Model file for the job. Use its own axes, mm. A direction names the side the tool comes from. Round coordinates to 2 decimals unless told otherwise and drop trailing zeros. Loops run counter-clockwise (first coordinate to the right, second up) from the corner with the lowest first, then second, coordinate; pieces in that order, holes last. Notation, with made-up numbers: M 86,43.25 L 143,43.25 A37 cw 143,79.25 Z; hole C 11,16.5 d9. An arc over 180 degrees is marked long. Use a Markdown table: item, result. Add a question column.
Item 1: Tool access for faces 5 (the flat face through (-44.25, 0.49, -44.49)), 6 (the flat face through (44.25, 0.51, -31.72)): list every direction of +Z, -Z, +X, -X, +Y, -Y with a clear straight run to the whole face (end or side of a thin tool).
Item 2: Saw through at A-A on z = 9.5. Write the cut outline in (x, y).
Item 3: Wall check: L1, parallel to Z at x = -38.5, y = 0.35; L2, parallel to Z at x = -10, y = 0.7; L3, parallel to Z at x = 3, y = 0.5. Give the ranges that are in metal, low to high. Write a range as from..to.
Item 4: Saw through at D-D on x = 50. Write the cut outline in (y, z).
Item 5: Saw through at B-B on x = -16.5. Write the cut outline in (y, z).
Item 6: Saw through at C-C on y = 0.8. Give the number of separate pieces and of enclosed holes in the cut face, then the cut area to 3 significant figures.
Item 7: Two-plate mould, pull along X, no slides. Class faces 1 (the flat face through (-24.17, 0.49, 57.91)), 2 (the flat face through (23.85, 0.49, 58.04)), 3 (the flat face through (44.25, 0.51, 31.72)), 4 (the flat face through (36.74, 0.493, -42.455)): +X half, -X half, draft (parallel to the pull), parting line (faces both ways), or undercut.
Item 8: Pin check, flat tip, straight feed: P1, Ø0.5, axis at x = 51.5, y = 0.5, coming from the +Z side. Stop position of the tip, or through.
```python
from build123d import *

# Parameters (mm, degrees)
BOSS_EXTRUDE1_DEPTH = 1
SKETCH2_W           = 10
SKETCH2_H           = 10
BOSS_EXTRUDE2_DEPTH = 1
SKETCH3_R           = 1.5
BOSS_EXTRUDE3_DEPTH = 1
CHAMFER1_SIZE       = 1.5


with BuildPart() as part:
    # Sketch1 → Boss-Extrude1 (new body)
    with BuildSketch(Plane(origin=(0, 0, 0), x_dir=(1, 0, 0), z_dir=(0, 1, 0))):
        Polygon((62.75, -12.481751053), (62.75, 12.481751053), (53.19688133, 35.545019709), (35.545019709, 53.19688133), (12.481751053, 62.75), (-12.481751053, 62.75), (-35.545019709, 53.19688133), (-53.19688133, 35.545019709), (-62.75, 12.481751053), (-62.75, -12.481751053), (-53.19688133, -35.545019709), (-35.545019709, -53.19688133), (-12.481751053, -62.75), (12.481751053, -62.75), (35.545019709, -53.19688133), (53.19688133, -35.545019709), align=None)
        Polygon((56, -11.139092573), (56, 11.139092573), (47.474507641, 31.721451852), (31.721451852, 47.474507641), (11.139092573, 56), (-11.139092573, 56), (-31.721451852, 47.474507641), (-47.474507641, 31.721451852), (-56, 11.139092573), (-56, -11.139092573), (-47.474507641, -31.721451852), (-31.721451852, -47.474507641), (-11.139092573, -56), (11.139092573, -56), (31.721451852, -47.474507641), (47.474507641, -31.721451852), align=None, mode=Mode.SUBTRACT)
    extrude(amount=BOSS_EXTRUDE1_DEPTH)

    # Sketch2 → Boss-Extrude2 (add)
    with BuildSketch(Plane(origin=(0, 1, 0), x_dir=(1, 0, 0), z_dir=(0, 1, 0))):
        with Locations((0, 51)):
            Rectangle(SKETCH2_W, SKETCH2_H)
        with Locations((51, 0)):
            Rectangle(SKETCH2_W, SKETCH2_H)
        with Locations((0, -51)):
            Rectangle(SKETCH2_W, SKETCH2_H)
        with Locations((-51, 0)):
            Rectangle(SKETCH2_W, SKETCH2_H)
    extrude(amount=-BOSS_EXTRUDE2_DEPTH)

    # Sketch3 → Boss-Extrude3 (add)
    # profile 1 of 4: a face of its own
    with BuildSketch(Plane(origin=(0, 1, 0), x_dir=(1, 0, 0), z_dir=(0, 1, 0))):
        Polygon((-45.863587475, 33.332372018), (-41.620946788, 37.575012705), (-37.378306101, 33.332372018), (-41.620946788, 29.08973133), align=None)
        with Locations(Location((-41.620946788, 33.332372018, 0), (0, 0, 270))):
            Circle(SKETCH3_R, mode=Mode.SUBTRACT)
    # profile 2 of 4: a face of its own
    with BuildSketch(Plane(origin=(0, 1, 0), x_dir=(1, 0, 0), z_dir=(0, 1, 0))):
        Polygon((37.378306101, 33.332372018), (41.620946788, 29.08973133), (45.863587475, 33.332372018), (41.620946788, 37.575012705), align=None)
        with Locations(Location((41.620946788, 33.332372018, 0), (0, 0, 270))):
            Circle(SKETCH3_R, mode=Mode.SUBTRACT)
    # profile 3 of 4: a face of its own
    with BuildSketch(Plane(origin=(0, 1, 0), x_dir=(1, 0, 0), z_dir=(0, 1, 0))):
        Polygon((41.620946788, -37.575012705), (37.378306101, -33.332372018), (41.620946788, -29.08973133), (45.863587475, -33.332372018), align=None)
        with Locations(Location((41.620946788, -33.332372018, 0), (0, 0, 270))):
            Circle(SKETCH3_R, mode=Mode.SUBTRACT)
    # profile 4 of 4: a face of its own
    with BuildSketch(Plane(origin=(0, 1, 0), x_dir=(1, 0, 0), z_dir=(0, 1, 0))):
        Polygon((-37.378306101, -33.332372018), (-41.620946788, -29.08973133), (-45.863587475, -33.332372018), (-41.620946788, -37.575012705), align=None)
        with Locations(Location((-41.620946788, -33.332372018, 0), (0, 0, 270))):
            Circle(SKETCH3_R, mode=Mode.SUBTRACT)
    extrude(amount=-BOSS_EXTRUDE3_DEPTH)

    # Chamfer1
    chamfer1_edges = [part.edges().sort_by_distance(p)[0] for p in [
        (-37.378306101, 0.5, -33.332372018),
        (-41.620946788, 0.5, -29.08973133),
        (41.620946788, 0.5, -29.08973133),
        (37.378306101, 0.5, -33.332372018),
        (41.620946788, 0.5, 29.08973133),
        (37.378306101, 0.5, 33.332372018),
        (-41.620946788, 0.5, 29.08973133),
        (-37.378306101, 0.5, 33.332372018),
    ]]
    chamfer(chamfer1_edges, length=CHAMFER1_SIZE)


solid = part.part
```
Entries:
| question | item | result |
|---|---|---|
| 1 | face 5 | -Z, -X, +Y, -Y |
| 1 | face 6 | +Y, -Y |
| 2 | outline | M -62.75,0 L -56,0 L -56,1 L -62.75,1 Z; M 56,0 L 62.75,0 L 62.75,1 L 56,1 Z |
| 3 | L1 | -50.24..-40.7, -34.45..-32.21, 32.21..34.45, 40.7..50.24 |
| 3 | L2 | -62.75..-56, 56..62.75 |
| 3 | L3 | -62.75..-46, 46..62.75 |
| 4 | outline | M 0,-38.74 L 1,-38.74 L 1,-25.62 L 0,-25.62 Z; M 0,-5 L 1,-5 L 1,5 L 0,5 Z; M 0,25.62 L 1,25.62 L 1,38.74 L 0,38.74 Z |
| 5 | outline | M 0,-61.09 L 1,-61.09 L 1,-53.78 L 0,-53.78 Z; M 0,53.78 L 1,53.78 L 1,61.09 L 0,61.09 Z |
| 6 | separate pieces | 1 |
| 6 | enclosed holes | 5 |
| 6 | area | 3,060 mm2 |
| 7 | face 1 | -X half |
| 7 | face 2 | +X half |
| 7 | face 3 | undercut |
| 7 | face 4 | undercut |
| 8 | P1 | z = 37.49 |
